```python
from build123d import *

# Parameters (mm, degrees)
SKETCH1_W           = 75.692
SKETCH1_H           = 15.24
BOSS_EXTRUDE1_DEPTH = 1.143
SKETCH2_R           = 0.508
BOSS_EXTRUDE2_DEPTH = 1.143


with BuildPart() as part:
    # Sketch1 → Boss-Extrude1 (new body)
    with BuildSketch(Plane.XY):
        Rectangle(SKETCH1_W, SKETCH1_H)
    extrude(amount=BOSS_EXTRUDE1_DEPTH)

    # Sketch2 → Boss-Extrude2 (add)
    with BuildSketch(Plane.XY.offset(1.143)):
        with BuildLine():
            Line((-3.81, -7.62), (3.81, -7.62))
            Line((3.81, -7.62), (3.81, -10.16))
            ThreePointArc((3.81, -10.16), (0, -13.97), (-3.81, -10.16))
            Line((-3.81, -10.16), (-3.81, -7.62))
        make_face()
        with Locations((0, -10.16)):
            Circle(SKETCH2_R, mode=Mode.SUBTRACT)
    extrude(amount=-BOSS_EXTRUDE2_DEPTH)


solid = part.part
```
Input: part model. Units: mm. Frame: model coordinates. Coordinates: 2 decimals unless noted, no trailing zeros. Order: outer loops, then holes, each group sorted by start corner. A loop starts at its lowest first (then second) coordinate and runs counter-clockwise, first axis right, second up. Notation, with made-up numbers: (55, 51.5) - (62, 51.5) arc R7 ccw to (62, 55.5) - close; hole circle Ø1 at (13.25, 51). An arc over 180 degrees is marked (long way). Put each result on its own line as item: value.
1. Contact query for a flat-ended pin moving along its axis: pin 1 Ø0.6 at (x, z) = (-15.5, 1) entering from -Y. Output: stop coordinate, or through.
Report:
pin 1: stops at y = -7.62
2. Cut plane B-B on x = -23. Return the cut outline in (y, z).
Report:
outline: (-7.62, 0) - (7.62, 0) - (7.62, 1.14) - (-7.62, 1.14) - close
3. Cut plane A-A on z = 0.7. Return the cut outline in (x, y), then the cut area to 3 significant figures.
Report:
outline: (-37.85, -7.62) - (-3.81, -7.62) - (-3.81, -10.16) arc R3.81 ccw to (3.81, -10.16) - (3.81, -7.62) - (37.85, -7.62) - (37.85, 7.62) - (-37.85, 7.62) - close; hole circle Ø1.02 at (0, -10.16)
area: 1,190 mm2
4. Draft query along Z for faces 1 (the face through (0.08, -13.97, 0.58)), 2 (the face through (-1, -1, 1.143)), 3 (the face through (-1, -1, 0)). Return one class per face: pulls with the +Z half, pulls with the -Z half, needs draft (parallel to the pull), parting line crosses it, or undercut.
Report:
face 1: needs draft
face 2: pulls with the +Z half
face 3: pulls with the -Z half
5. Line query: line 1 along Y through (x, z) = (0, 0.6); line 2 along X through (y, z) = (-7.75, 0.1); line 3 along Y through (x, z) = (6, 0.45). Output: solid intervals per line, ascending.
Report:
line 1: y = -13.97 to -10.67, -9.65 to 7.62
line 2: x = -3.81 to 3.81
line 3: y = -7.62 to 7.62
